Verification items for the finished model (mm, model axes). Face numbers are marked on the shaded views. A direction names the side the tool comes from. Coordinates: 2 decimals unless noted, no trailing zeros. Write each loop counter-clockwise with the first axis right and the second up, starting at its lowest first coordinate (ties: lowest second). Pieces come first, ordered by that corner, then holes.
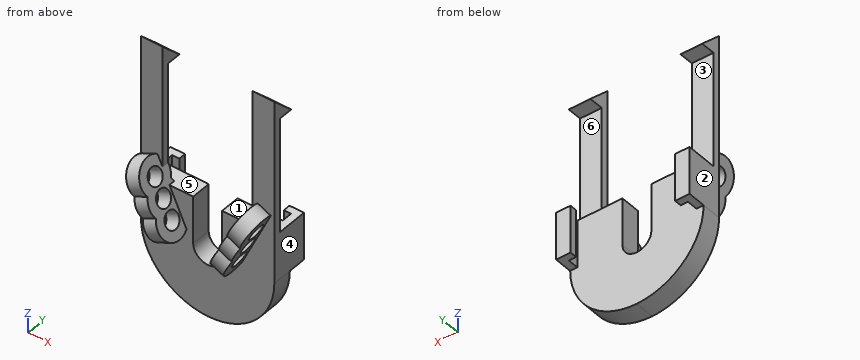
```python
from build123d import *

# Parameters (mm, degrees)
SKETCH002_R  = 2.35
PAD005_DEPTH = 4
PAD002_DEPTH = 8
PAD001_DEPTH = 5.5
PAD_DEPTH    = 13.2
SKETCH005_W  = 6
SKETCH005_H  = 2
PAD003_DEPTH = 38
PAD004_DEPTH = 6
POCKET_DEPTH = 6


with BuildPart() as pad005:
    # Sketch002 → Pad005 (new body)
    with BuildSketch(Plane(origin=(5, -3, 10), x_dir=(0.422618, 0, -0.906308), z_dir=(0.906308, 0, 0.422618))):
        with BuildLine():
            ThreePointArc((-2.75, 4.175823), (-10.5, 0), (-2.75, -4.175823))
            ThreePointArc((-2.75, -4.175823), (0, -5), (2.75, -4.175823))
            ThreePointArc((2.75, -4.175823), (10.5, 0), (2.75, 4.175823))
            ThreePointArc((2.75, 4.175823), (0, 5), (-2.75, 4.175823))
        make_face()
        with Locations((-5.5, 0)):
            Circle(SKETCH002_R, mode=Mode.SUBTRACT)
        Circle(SKETCH002_R, mode=Mode.SUBTRACT)
        with Locations((5.5, 0)):
            Circle(SKETCH002_R, mode=Mode.SUBTRACT)
    extrude(amount=PAD005_DEPTH)


with BuildPart() as pad002:
    # Sketch004 → Pad002 (new body)
    with BuildSketch(Plane.XZ):
        with BuildLine():
            Line((14.5, 20), (18.5, 20))
            Line((18.5, 20), (18.5, -4))
            ThreePointArc((14.5, 1.7e-05), (15.671567, -2.828421), (18.5, -4))
            Line((14.5, 20), (14.5, 1.7e-05))
        make_face()
    extrude(amount=-PAD002_DEPTH)


with BuildPart() as pad001:
    # Sketch001 → Pad001 (new body)
    with BuildSketch(Plane.XZ):
        with BuildLine():
            ThreePointArc((0, 0), (5.418525, -13.081475), (18.5, -18.5))
            Line((18.5, 0), (18.5, -18.5))
            Line((18.5, 0), (0, 0))
        make_face()
    extrude(amount=-PAD001_DEPTH)


with BuildPart() as fusion001:
    # Sketch → Pad (new body)
    with BuildSketch(Plane.XY):
        Polygon((2, 5.5), (18.5, 5.5), (18.5, 0), (0, 0), (0, 10.5), (4, 10.5), (4, 8.5), (2, 8.5), align=None)
    extrude(amount=PAD_DEPTH)

    # Fusion: union Pad001
    add(pad001.part)

    # Cut: cut Pad002
    add(pad002.part, mode=Mode.SUBTRACT)

    # Sketch005 → Pad003 (new body)
    with BuildSketch(Plane.XY.offset(13.2)):
        with Locations((3, 1)):
            Rectangle(SKETCH005_W, SKETCH005_H)
    extrude(amount=PAD003_DEPTH)

    # Sketch006 → Pad004 (new body)
    with BuildSketch(Plane(origin=(0, 0, 0), x_dir=(0, -1, 0), z_dir=(-1, 0, 0))):
        Polygon((0, 51.2), (0, 45.2), (-6, 45.2), align=None)
    extrude(amount=-PAD004_DEPTH)

    # Sketch007 → Pocket (cut)
    with BuildSketch(Plane(origin=(0, 0, 0), x_dir=(0, -1, 0), z_dir=(-1, 0, 0))):
        Polygon((-2, 51.2), (0, 51.2), (-2, 49.2), align=None)
    extrude(amount=-POCKET_DEPTH, mode=Mode.SUBTRACT)

    # Fusion001: union Pad005
    add(pad005.part)


with BuildPart() as part_mirroring:
    # Part__Mirroring: instance of Fusion001
    add(fusion001.part.mirror(Plane(origin=(0, 0, 0), x_dir=(0, -1, 0), z_dir=(1, 0, 0))))


with BuildPart() as part_mirroring_1:
    # Part__Mirroring placement: moved
    add(part_mirroring.part.moved(Location((37, 0, 0))))


with BuildPart() as fusion002:
    # Fusion002 base: copy of Fusion001
    add(fusion001.part)

    # Fusion002: union Part__Mirroring
    add(part_mirroring_1.part)


solid = fusion002.part
```
1. Material ranges on L1, parallel to X at y = 5, z = 3; L2, parallel to Z at x = 4.5, y = -4; L3, parallel to Y at x = 10.5, z = 5, recorded low to high.
2. Sectioned sample at A-A, the plane y = 3.75. Record the boundary of the cut face in (x, z), and give its area (3 significant figures).
3. Sectioned sample at C-C, the plane y = -4.5. Give the number of separate pieces and of enclosed holes in the cut face, and give its area (3 significant figures).
4. Tool access check on the marked faces 1, 2 and 3. Record the directions out of +Z, -Z, +X, -X, +Y, -Y that give a thin tool (end or side, any length) a straight path to the whole face; none if there is none.
5. Draft check along X on the marked faces 4, 5 and 6. Enter one of: pulls with the +X half, pulls with the -X half, needs draft (parallel to the pull), parting line crosses it, or undercut.
6. Sectioned sample at D-D, the plane z = -11. Record the boundary of the cut face in (x, y), and give its area (3 significant figures).
7. Sectioned sample at B-B, the plane z = 32. Record the boundary of the cut face in (x, y), and give its area (3 significant figures).
8. Gauge pin test, flat ends, axial feed: P1, Ø2, axis at x = 2.5, y = 3, coming from the -Z side; P2, Ø4.5, axis at x = 34.5, y = 8, coming from the -Z side; P3, Ø3, axis at x = 3.5, z = 29.5, coming from the +Y side; P4, Ø6, axis at y = 7.5, z = 40.5, coming from the -X side. Record the tip position at first contact, or that the pin passes through.
Outcome:
1. L1: x = 0 to 14.5, 22.5 to 37
1. L2: z = 12.11 to 13.49, 18.18 to 20.54
1. L3: y = -7.81 to -4.92, -1.08 to 5.5
2. outline: (0, 0) arc R18.5 ccw to (18.5, -18.5) arc R18.5 ccw to (37, 0) - (37, 13.2) - (22.5, 13.2) - (22.5, 0) arc R4 cw to (14.5, 0) - (14.5, 13.2) - (0, 13.2) - close; (0, 45.2) - (6, 45.2) - (6, 47.45) - (0, 47.45) - close; (31, 45.2) - (37, 45.2) - (37, 47.45) - (31, 47.45) - close
2. area: 922 mm2
3. separate pieces: 8
3. enclosed holes: 0
3. area: 77.5 mm2
4. face 1: +Y
4. face 2: +Z, -Z, -X, +Y, -Y
4. face 3: +X, -X, +Y
5. face 4: pulls with the +X half
5. face 5: undercut
5. face 6: needs draft
6. outline: (3.63, 0) - (33.37, 0) - (33.37, 5.5) - (3.63, 5.5) - close
6. area: 164 mm2
7. outline: (0, 0) - (6, 0) - (6, 2) - (0, 2) - close; (31, 0) - (37, 0) - (37, 2) - (31, 2) - close
7. area: 24.0 mm2
8. P1: stops at z = -10.83
8. P2: stops at z = 0
8. P3: stops at y = 2
8. P4: passes through
